from build123d import *

# Parameters (mm, degrees)
F0_W           = 50.8
F0_H           = 50.8
F1_DEPTH       = 25.4
F1_DEPTH_BACK  = 25.4
F2_W           = 25.4
F2_H           = 25.4
F3_DEPTH       = 12.7
F3_DEPTH_BACK  = 12.7
F6_DEPTH       = 12.7
F6_DEPTH_BACK  = 12.7
F9_DEPTH       = 12.7
F9_DEPTH_BACK  = 12.7
F11_DEPTH      = 5.08
F11_DEPTH_BACK = 10.16
F16_SIZE       = 5.08
F17_SIZE       = 5.08


with BuildPart() as f1:
    # F0 (on Front) → F1 (new body, two sides)
    with BuildSketch(Plane.XZ) as f1_sk:
        Rectangle(F0_W, F0_H)
    extrude(amount=F1_DEPTH)
    extrude(f1_sk.sketch, amount=-F1_DEPTH_BACK)

    # F2 (on face) → F3 (join, two sides)
    with BuildSketch(Plane.XZ.offset(25.4)) as f3_sk:
        with Locations((-25.4, 25.4)):
            Rectangle(F2_W, F2_H)
        with Locations((25.4, 25.4)):
            Rectangle(F2_W, F2_H)
        with Locations((25.4, -25.4)):
            Rectangle(F2_W, F2_H)
        with Locations((-25.4, -25.4)):
            Rectangle(F2_W, F2_H)
        Polygon((17.9605122421, 0), (0, 17.9605122421), (-17.9605122421, 0), (0, -17.9605122421), align=None)
    extrude(amount=F3_DEPTH)
    extrude(f3_sk.sketch, amount=-F3_DEPTH_BACK)

    # F4: F1 across plane


with BuildPart() as f1_1:
    add(f1.part)
    add(f1.part.mirror(Plane.XZ))

    # F5 (on face) → F6 (join, two sides)
    with BuildSketch(Plane(origin=(0, 0, -25.4), x_dir=(1, 0, 0), z_dir=(0, 0, -1))) as f6_sk:
        Polygon((17.9605122421, 0), (0, 17.9605122421), (-17.9605122421, 0), (0, -17.9605122421), align=None)
    extrude(amount=F6_DEPTH)
    extrude(f6_sk.sketch, amount=-F6_DEPTH_BACK)

    # F7: F1 across plane


with BuildPart() as f1_2:
    add(f1_1.part)
    add(f1_1.part.mirror(Plane.XY))

    # F8 (on face) → F9 (join, two sides)
    with BuildSketch(Plane(origin=(-25.4, 0, 0), x_dir=(0, -1, 0), z_dir=(-1, 0, 0))) as f9_sk:
        Polygon((17.9605122421, 0), (0, 17.9605122421), (-17.9605122421, 0), (0, -17.9605122421), align=None)
    extrude(amount=F9_DEPTH)
    extrude(f9_sk.sketch, amount=-F9_DEPTH_BACK)

    # F10 (on face) → F11 (join, two sides)
    with BuildSketch(Plane(origin=(-38.1, 0, 0), x_dir=(0, -1, 0), z_dir=(-1, 0, 0))) as f11_sk:
        Polygon((-38.1, -38.1), (-38.1, -25.4), (-41.402, -25.4), (-41.402, -38.1), (-41.402, -41.402), (-38.1, -41.402), (-25.4, -41.402), (-25.4, -38.1), align=None)
        with BuildLine():
            Line((-31.75, -25.4), (-38.1, -25.4))
            Line((-38.1, -25.4), (-38.1, -38.1))
            Line((-38.1, -38.1), (-25.4, -38.1))
            Line((-25.4, -38.1), (-25.4, -31.75))
            ThreePointArc((-25.4, -31.75), (-29.8901280605, -29.8901280605), (-31.75, -25.4))
        make_face()
    extrude(amount=F11_DEPTH)
    extrude(f11_sk.sketch, amount=-F11_DEPTH_BACK)

    # F12: F1 across plane


with BuildPart() as f1_3:
    add(f1_2.part)
    add(f1_2.part.mirror(Plane.YZ))

    # F13: F1 across plane


with BuildPart() as f1_4:
    add(f1_3.part)
    add(f1_3.part.mirror(Plane.XY))

    # F14: F1 across plane


with BuildPart() as f1_5:
    add(f1_4.part)
    add(f1_4.part.mirror(Plane.XZ))

    # F15: F1 across plane


with BuildPart() as f1_6:
    add(f1_5.part)
    add(f1_5.part.mirror(Plane.YZ), mode=Mode.INTERSECT)

    # F16
    f16_edges = [f1_6.edges().sort_by_distance(p)[0] for p in [
        (12.7, 12.7, -31.75),
        (12.7, -12.7, -31.75),
        (-12.7, -12.7, -31.75),
        (-12.7, 12.7, -31.75),
        (-12.7, 31.75, -12.7),
        (12.7, 31.75, 12.7),
        (-12.7, 31.75, 12.7),
        (31.75, 12.7, 12.7),
        (31.75, -12.7, 12.7),
        (31.75, -12.7, -12.7),
        (31.75, 12.7, -12.7),
        (-12.7, -12.7, 31.75),
        (-12.7, 12.7, 31.75),
        (12.7, -31.75, 12.7),
        (-12.7, -31.75, -12.7),
        (12.7, -31.75, -12.7),
        (12.7, 12.7, 31.75),
        (12.7, -12.7, 31.75),
        (-31.75, 12.7, -12.7),
        (-31.75, 12.7, 12.7),
        (-31.75, -12.7, -12.7),
        (-31.75, -12.7, 12.7),
        (-12.7, -31.75, 12.7),
    ]]
    chamfer(f16_edges, length=F16_SIZE)

    # F17
    f17_edges = [f1_6.edges().sort_by_distance(p)[0] for p in [
        (-38.1, 8.980256, -8.980256),
        (-38.1, -8.980256, -8.980256),
        (-38.1, -8.980256, 8.980256),
        (-38.1, 8.980256, 8.980256),
        (8.980256, -8.980256, -38.1),
        (-8.980256, -8.980256, -38.1),
        (-8.980256, 8.980256, -38.1),
        (8.980256, 8.980256, -38.1),
        (8.980256, 38.1, 8.980256),
        (-8.980256, 38.1, 8.980256),
        (-8.980256, 38.1, -8.980256),
        (8.980256, 38.1, -8.980256),
        (8.980256, -8.980256, 38.1),
        (-8.980256, -8.980256, 38.1),
        (-8.980256, 8.980256, 38.1),
        (8.980256, 8.980256, 38.1),
        (38.1, 8.980256, -8.980256),
        (38.1, -8.980256, -8.980256),
        (38.1, -8.980256, 8.980256),
        (38.1, 8.980256, 8.980256),
        (8.980256, -38.1, 8.980256),
        (-8.980256, -38.1, 8.980256),
        (-8.980256, -38.1, -8.980256),
        (8.980256, -38.1, -8.980256),
    ]]
    chamfer(f17_edges, length=F17_SIZE)


solid = f1_6.part
Geometry: final body of the model. Coordinates: model frame, mm. A direction names the side the tool comes from. Round coordinates to 2 decimals unless told otherwise and drop trailing zeros. Loops run counter-clockwise (first coordinate to the right, second up) from the corner with the lowest first, then second, coordinate; pieces in that order, holes last.
Q1. Section B-B on x = -31.5. State how many separate pieces and enclosed holes the cut face has, plus the area to 3 significant figures.
Q2. Section D-D on x = -8.5. Return loops of the section in (y, z).
Q3. Material intervals for L1, parallel to X at y = -28.5, z = 25; L2, parallel to Z at x = -32, y = -31.5, sorted ascending.
Q4. Pull-direction query (Z, two-part tool) for faces 4 (the flat face through (-8.85, -29.16, 9.11)), 5 (the flat face through (36, -34, 41.402)), 6 (the flat face through (-12.7, 28, 28)), 7 (the flat face through (38.1, -22, -23)); classes: released by +Z, released by -Z, zero draft, split by the parting line, or undercut.
Q5. Access query for faces 1 (the flat face through (9.11, 29.16, 8.85)), 2 (the flat face through (-28, 28, -12.7)), 3 (the cylindrical face through (-40.6, -29.84, -29.94)). Directions: +Z, -Z, +X, -X, +Y, -Y. A direction counts if a zero-diameter tool reaches every point of the face in a straight line with its end or side. Return the directions, or none.
Q6. Section A-A on z = 21.5. Return loops of the section in (x, y).
Q7. Pin query (flat end, axial travel): P1, Ø2, axis at x = 17.5, z = 12.5, coming from the +Y side; P2, Ø8, axis at x = -2, y = -24, coming from the +Z side; P3, Ø4, axis at x = -21.5, y = -8, coming from the -Z side. Return the tip coordinate at first contact, or that it passes through.
Evaluation:
1. separate pieces: 5
1. enclosed holes: 0
1. area: 3,550 mm2
2. outline: (-38.1, -2.28) - (-33.02, -9.46) - (-25.4, -9.46) - (-25.4, -25.4) - (-9.46, -25.4) - (-9.46, -33.02) - (-2.28, -38.1) - (2.28, -38.1) - (9.46, -33.02) - (9.46, -25.4) - (25.4, -25.4) - (25.4, -9.46) - (33.02, -9.46) - (38.1, -2.28) - (38.1, 2.28) - (33.02, 9.46) - (25.4, 9.46) - (25.4, 25.4) - (9.46, 25.4) - (9.46, 33.02) - (2.28, 38.1) - (-2.28, 38.1) - (-9.46, 33.02) - (-9.46, 25.4) - (-25.4, 25.4) - (-25.4, 9.46) - (-33.02, 9.46) - (-38.1, 2.28) - close
3. L1: x = -38.1 to -12.7, 12.7 to 38.1
3. L2: z = -41.4 to -12.7, 12.7 to 41.4
4. face 4: undercut
4. face 5: released by +Z
4. face 6: zero draft
4. face 7: undercut
5. face 1: +Y
5. face 2: -X, +Y
5. face 3: -X
6. outline: (-38.1, -38.1) - (-12.7, -38.1) - (-12.7, -25.4) - (12.7, -25.4) - (12.7, -38.1) - (38.1, -38.1) - (38.1, -12.7) - (25.4, -12.7) - (25.4, 12.7) - (38.1, 12.7) - (38.1, 38.1) - (12.7, 38.1) - (12.7, 25.4) - (-12.7, 25.4) - (-12.7, 38.1) - (-38.1, 38.1) - (-38.1, 12.7) - (-25.4, 12.7) - (-25.4, -12.7) - (-38.1, -12.7) - close
7. P1: stops at y = 38.1
7. P2: stops at z = 25.4
7. P3: stops at z = -25.4
